The listing builds one solid part. Answer for the finished solid, in the listing's coordinates (mm). A direction names the side the tool comes from. Coordinates: 2 decimals unless noted, no trailing zeros. Write each loop counter-clockwise with the first axis right and the second up, starting at its lowest first coordinate (ties: lowest second). Pieces come first, ordered by that corner, then holes.
Autodesk Inventor part; units mm, degrees
ref_plane "Start plane" through (0, 0, 0) normal (0, 0, 1) x (1, 0, 0)
ref_plane "End plane" through (0, 0, 2800) normal (0, 0, 1) x (1, 0, 0)
ref_plane "YZ Plane" through (0, 0, 0) normal (1, 0, 0) x (0, 1, 0)
ref_plane "Start plane" through (0, 0, 0) normal (0, 0, 1) x (1, 0, 0)
ref_plane "End plane" through (0, 0, 2800) normal (0, 0, 1) x (1, 0, 0)
sketch "Sketch" plane through (0, 0, 0) normal (0, 0, 1) x (1, 0, 0)
  line L0 (-20, -24) -> (-20, 24)
  line L1 (-14, 30) -> (14, 30)
  line L2 (20, 24) -> (20, -24)
  line L3 (14, -30) -> (-14, -30)
  arc A0 (-20, -24) -> (-14, -30) centre (-14, -24) ccw
  arc A1 (20, 24) -> (14, 30) centre (14, 24) ccw
  arc A2 (-14, 30) -> (-20, 24) centre (-14, 24) ccw
  arc A3 (14, -30) -> (20, -24) centre (14, -24) ccw
  arc A4 (-14, 27) -> (-17, 24) centre (-14, 24) ccw
  line L4 (-14, 27) -> (14, 27)
  arc A5 (17, 24) -> (14, 27) centre (14, 24) ccw
  line L5 (17, 24) -> (17, -24)
  arc A6 (14, -27) -> (17, -24) centre (14, -24) ccw
  line L6 (14, -27) -> (-14, -27)
  arc A7 (-17, -24) -> (-14, -27) centre (-14, -24) ccw
  line L7 (-17, -24) -> (-17, 24)
  line L8 (0, 43.7397) -> (0, -43.7397) construction
  line L9 (-29.7397, 0) -> (29.7397, 0) construction
  dimension "d7" = 6
  dimension "d9" = 40
  dimension "d11" = 60
  dimension "d12" = 3
  dimension "d15" = 20
  dimension "d16" = 30
extrude "Body" add sketch "Sketch" along normal up to surface (2800 mm away) from surface at 0
sketch "Sketch3" plane through (0, 0, 0) normal (0, 0, 1) x (1, 0, 0)
  line L0 (0, 0) -> (10, 0)
ref_plane "Work Plane3" through (0, 0, 0) normal (0, -1, 0) x (1, 0, 0)
sketch "Sketch7" plane through (0, 0, 0) normal (1, 0, 0) x (0, 1, 0)
  line L0 (-30, 0) -> (-30, 2800)
  line L1 (-30, 0) -> (-30, 2800)
  line L2 (30, 0) -> (30, 2800)
  line L3 (30, 0) -> (30, 2800)
  line L4 (-30, 0) -> (-24, 0)
  line L5 (30, 0) -> (-30, 0)
  line L6 (30, 0) -> (-30, 60)
  line L7 (-30, 0) -> (-30, 2800)
  line L8 (30, 2800) -> (-30, 2800)
  line L9 (-30, 2800) -> (30, 2740)
  point P0 (0, 0)
  dimension "d26" = 45
  dimension "d27" = 45
extrude "Extrusion4" cut sketch "Sketch7" along normal through all both and the other way through all contours L0 L6 L5 L4 | L8 L2 L9
sketch "Sketch4" plane through (0, 0, 0) normal (0, -1, 0) x (1, 0, 0)
  line L0 (-2, 0) -> (12, 0)
  line L1 (-2, 2800) -> (12, 2800)
  dimension "d18" = 2800
equation "\"d7\" = G_IR"
equation "\"d9\" = G_W"
equation "\"d11\" = G_H"
equation "\"d12\" = G_T"
equation "\"d15\" = 0.5 * d9"
equation "\"d16\" = 0.5 * d11"
equation "\"d3\" = G_L"
equation "\"G_W\" = 40"
equation "\"G_H\" = 60"
equation "\"G_T\" = 3"
equation "\"G_IR\" = 6"
equation "\"G_L\" = d18"
equation "\"G_OFFSET_START\" = 0"
equation "\"G_OFFSET_END\" = 0"
properties part number "ISO 4019 - 60x40x3 - 2800" material "Steel, Mild"
1. Find the intervals of material crossed by L1, parallel to Y at x = 9.5, z = 334; L2, parallel to X at y = -21.5, z = 2228; L3, parallel to Y at x = -15.5, z = 772.5, in increasing order.
Results found:
L1: y = -30 to -27, 27 to 30
L2: x = -20 to -17, 17 to 20
L3: y = -29.81 to -26.6, 26.6 to 29.81
2. A tool of negligible diameter and unlimited length cuts with its end or side. For faces 1 (the flat face through (20, 0, 1380)), 2 (the flat face through (17, 0, 1380)), from which of +Z, -Z, +X, -X, +Y, -Y can it reach the whole face along a straight path? Write none if from no direction.
Results found:
face 1: +Z, -Z, +X, +Y, -Y
face 2: +Z, -Z
3. A flat-ended cylindrical pin translates along its axis: P1, Ø3, axis at x = -16, y = 21, coming from the +Z side. Find the tip coordinate at first contact, or state that the pin passes through.
Results found:
P1: stops at z = 2750.12
4. For a pull along Y with two mould halves and no side action, classify faces 3 (the flat face through (18, 0, 2770)), 4 (the flat face through (-17, 0, 1380)), 5 (the flat face through (-20, 0, 1380)), 6 (the flat face through (18, 0, 30)) as pulls with the +Y half, pulls with the -Y half, needs draft (parallel to the pull), parting line crosses it, or undercut.
Results found:
face 3: pulls with the +Y half
face 4: undercut
face 5: needs draft
face 6: pulls with the -Y half
5. Section B-B on x = -2 is taken. Give the vertices of the cut face in (y, z), then the cut area to 3 significant figures.
Results found:
outline: (-30, 60) - (-27, 57) - (-27, 2797) - (-30, 2800) - close; (27, 3) - (30, 0) - (30, 2740) - (27, 2743) - close
area: 16,400 mm2
6. Section A-A on y = 7 is taken. Give the vertices of the cut face in (x, z).
Results found:
outline: (-20, 23) - (-17, 23) - (-17, 2763) - (-20, 2763) - close; (17, 23) - (20, 23) - (20, 2763) - (17, 2763) - close
7. Section C-C on z = 2300.5 is taken. Give the vertices of the cut face in (x, y).
Results found:
outline: (-20, -24) arc R6 ccw to (-14, -30) - (14, -30) arc R6 ccw to (20, -24) - (20, 24) arc R6 ccw to (14, 30) - (-14, 30) arc R6 ccw to (-20, 24) - close; hole (-17, -24) arc R3 ccw to (-14, -27) - (14, -27) arc R3 ccw to (17, -24) - (17, 24) arc R3 ccw to (14, 27) - (-14, 27) arc R3 ccw to (-17, 24) - close
